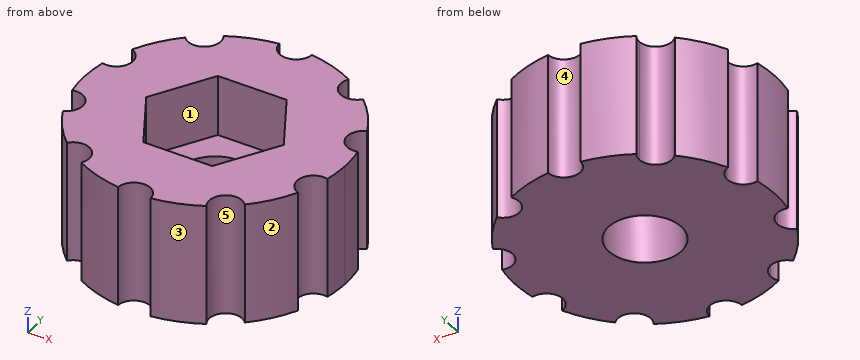
from build123d import *

# Parameters (mm, degrees)
F1_DEPTH = 10
F2_R     = 3
F3_DEPTH = 10.001
F4_R     = 3
F5_DEPTH = 5


with BuildPart() as f1:
    # F0 (on Top) → F1 (new body)
    with BuildSketch(Plane.XY):
        with BuildLine():
            ThreePointArc((10.6036903919, -2.023307953), (10.747066176, -1.0161661329), (10.795, 0))
            ThreePointArc((10.795, 0), (10.747066176, 1.0161661329), (10.6036903919, 2.023307953))
            ThreePointArc((10.6036903919, 2.023307953), (8.9778667931, 2.9170857512), (9.7678363058, 4.5958023134))
            ThreePointArc((9.7678363058, 4.5958023134), (8.7333384543, 6.3451417985), (7.3892951545, 7.8695833511))
            ThreePointArc((7.3892951545, 7.8695833511), (5.5486268246, 7.6370296448), (5.2010007473, 9.4594723017))
            ThreePointArc((5.2010007473, 9.4594723017), (3.3358384543, 10.2666550934), (1.352440321, 10.7099453863))
            ThreePointArc((1.352440321, 10.7099453863), (0, 9.4398877872), (-1.352440321, 10.7099453863))
            ThreePointArc((-1.352440321, 10.7099453863), (-3.3358384543, 10.2666550934), (-5.2010007473, 9.4594723017))
            ThreePointArc((-5.2010007473, 9.4594723017), (-5.0438407916, 9.1114188675), (-4.9900295857, 8.7333384543))
            ThreePointArc((-4.9900295857, 8.7333384543), (-5.8861297374, 7.4583337339), (-7.3892951545, 7.8695833511))
            ThreePointArc((-7.3892951545, 7.8695833511), (-8.7333384543, 6.3451417985), (-9.7678363058, 4.5958023134))
            ThreePointArc((-9.7678363058, 4.5958023134), (-9.1458775641, 4.0975384208), (-8.9115428806, 3.3358384543))
            ThreePointArc((-8.9115428806, 3.3358384543), (-9.4361105551, 2.2650794341), (-10.6036903919, 2.023307953))
            ThreePointArc((-10.6036903919, 2.023307953), (-10.795, 0), (-10.6036903919, -2.023307953))
            ThreePointArc((-10.6036903919, -2.023307953), (-9.4361105551, -2.2650794341), (-8.9115428806, -3.3358384543))
            ThreePointArc((-8.9115428806, -3.3358384543), (-9.1458775641, -4.0975384208), (-9.7678363058, -4.5958023134))
            ThreePointArc((-9.7678363058, -4.5958023134), (-8.7333384543, -6.3451417985), (-7.3892951545, -7.8695833511))
            ThreePointArc((-7.3892951545, -7.8695833511), (-5.8861297374, -7.4583337339), (-4.9900295857, -8.7333384543))
            ThreePointArc((-4.9900295857, -8.7333384543), (-5.0438407916, -9.1114188675), (-5.2010007473, -9.4594723017))
            ThreePointArc((-5.2010007473, -9.4594723017), (-3.3358384543, -10.2666550934), (-1.352440321, -10.7099453863))
            ThreePointArc((-1.352440321, -10.7099453863), (0, -9.4398877872), (1.352440321, -10.7099453863))
            ThreePointArc((1.352440321, -10.7099453863), (3.3358384543, -10.2666550934), (5.2010007473, -9.4594723017))
            ThreePointArc((5.2010007473, -9.4594723017), (5.5486268246, -7.6370296448), (7.3892951545, -7.8695833511))
            ThreePointArc((7.3892951545, -7.8695833511), (8.7333384543, -6.3451417985), (9.7678363058, -4.5958023134))
            ThreePointArc((9.7678363058, -4.5958023134), (8.9778667931, -2.9170857512), (10.6036903919, -2.023307953))
        make_face()
    extrude(amount=F1_DEPTH)

    # F2 (on face) → F3 (cut, through all)
    with BuildSketch(Plane.XY.offset(10)):
        Circle(F2_R)
    extrude(amount=-F3_DEPTH, mode=Mode.SUBTRACT)

    # F4 (on face) → F5 (cut)
    with BuildSketch(Plane.XY.offset(10)):
        Polygon((2.8578838325, -4.95), (5.715767665, 0), (2.8578838325, 4.95), (-2.8578838325, 4.95), (-5.715767665, 0), (-2.8578838325, -4.95), align=None)
        Circle(F4_R, mode=Mode.SUBTRACT)
    extrude(amount=-F5_DEPTH, mode=Mode.SUBTRACT)


solid = f1.part
Model file for the job. Use its own axes, mm. Face numbers are marked on the shaded views. A direction names the side the tool comes from. Give positions to 0.01 mm unless a question says otherwise; leave off trailing zeros. Loops run counter-clockwise (first coordinate to the right, second up) from the corner with the lowest first, then second, coordinate; pieces in that order, holes last.
1) Saw through at C-C (y = 1.25). Write the cut outline in (x, z).
2) Wall check: line 1 (Y direction, x = 0, z = 2.2); line 2 (Y direction, x = -0.25, z = 3.5); line 3 (X direction, y = 3.25, z = 8.5). Give the ranges that are in metal, low to high.
3) Saw through at A-A (z = 2). Write the cut outline in (x, y) (3 decimals).
4) Flat gauge pins, fed straight in: pin 1 Ø1 at (x, z) = (6.5, 6) entering from +Y; pin 2 Ø1 at (x, z) = (2.5, 3.5) entering from -Y; pin 3 Ø7 at (x, y) = (0, 0) entering from +Z. Where does each tip first touch, or does it go through?
5) Tool access for the marked faces 1 and 2: list every direction of +Z, -Z, +X, -X, +Y, -Y with a clear straight run to the whole face (end or side of a thin tool).
6) Saw through at B-B (x = 0). Write the cut outline in (y, z).
7) Pull direction Y, two halves, no side cores. Call the marked faces 3, 4 and 5: +Y half, -Y half, draft (parallel to the pull), parting line (faces both ways), or undercut.
8) Saw through at D-D (z = 7.5). Write the cut outline in (x, y) (3 decimals).
Answer block:
1. outline: (-10.72, 0) - (-2.73, 0) - (-2.73, 5) - (-4.99, 5) - (-4.99, 10) - (-10.72, 10) - close; (2.73, 0) - (10.72, 0) - (10.72, 10) - (4.99, 10) - (4.99, 5) - (2.73, 5) - close
2. line 1: y = -9.44 to -3, 3 to 9.44
2. line 2: y = -9.46 to -2.99, 2.99 to 9.46
2. line 3: x = -8.91 to -3.84, 3.84 to 8.91
3. outline: (-10.604, -2.023) arc R1.355 cw to (-9.768, -4.596) arc R10.795 ccw to (-7.389, -7.87) arc R1.355 cw to (-5.201, -9.459) arc R10.795 ccw to (-1.352, -10.71) arc R1.355 cw to (1.352, -10.71) arc R10.795 ccw to (5.201, -9.459) arc R1.355 cw to (7.389, -7.87) arc R10.795 ccw to (9.768, -4.596) arc R1.355 cw to (10.604, -2.023) arc R10.795 ccw to (10.604, 2.023) arc R1.355 cw to (9.768, 4.596) arc R10.795 ccw to (7.389, 7.87) arc R1.355 cw to (5.201, 9.459) arc R10.795 ccw to (1.352, 10.71) arc R1.355 cw to (-1.352, 10.71) arc R10.795 ccw to (-5.201, 9.459) arc R1.355 cw to (-7.389, 7.87) arc R10.795 ccw to (-9.768, 4.596) arc R1.355 cw to (-10.604, 2.023) arc R10.795 ccw to start; hole circle Ø6 at (0, 0)
4. pin 1: stops at y = 7.55
4. pin 2: stops at y = -10.61
4. pin 3: stops at z = 5
5. face 1: +Z
5. face 2: +Z, -Z, +X, -Y
6. outline: (-9.44, 0) - (-3, 0) - (-3, 5) - (-4.95, 5) - (-4.95, 10) - (-9.44, 10) - close; (3, 0) - (9.44, 0) - (9.44, 10) - (4.95, 10) - (4.95, 5) - (3, 5) - close
7. face 3: -Y half
7. face 4: +Y half
7. face 5: undercut
8. outline: (-10.604, -2.023) arc R1.355 cw to (-9.768, -4.596) arc R10.795 ccw to (-7.389, -7.87) arc R1.355 cw to (-5.201, -9.459) arc R10.795 ccw to (-1.352, -10.71) arc R1.355 cw to (1.352, -10.71) arc R10.795 ccw to (5.201, -9.459) arc R1.355 cw to (7.389, -7.87) arc R10.795 ccw to (9.768, -4.596) arc R1.355 cw to (10.604, -2.023) arc R10.795 ccw to (10.604, 2.023) arc R1.355 cw to (9.768, 4.596) arc R10.795 ccw to (7.389, 7.87) arc R1.355 cw to (5.201, 9.459) arc R10.795 ccw to (1.352, 10.71) arc R1.355 cw to (-1.352, 10.71) arc R10.795 ccw to (-5.201, 9.459) arc R1.355 cw to (-7.389, 7.87) arc R10.795 ccw to (-9.768, 4.596) arc R1.355 cw to (-10.604, 2.023) arc R10.795 ccw to start; hole (-5.716, 0) - (-2.858, -4.95) - (2.858, -4.95) - (5.716, 0) - (2.858, 4.95) - (-2.858, 4.95) - close
